Autodesk Inventor part; units mm, degrees
ref_plane "YZ Plane" through (0, 0, 0) normal (1, 0, 0) x (0, 1, 0)
ref_plane "XZ Plane" through (0, 0, 0) normal (0, 1, 0) x (-1, 0, 0)
ref_plane "XY Plane" through (0, 0, 0) normal (0, 0, 1) x (1, 0, 0)
sketch "Esboço1" plane through (0, 0, 0) normal (0, 1, 0) x (-1, 0, 0)
  line L0 (0, 0) -> (40, 0)
  line L1 (40, 0) -> (40, -60)
  line L2 (40, -60) -> (0, -60)
  line L3 (0, -60) -> (0, 0)
  dimension "d0" = 40
  dimension "d1" = 60
extrude "Extrusão1" add sketch "Esboço1" along normal blind 5
chamfer "Chanfro1" distance 3 angle 45 4 edges at (0, 2.5, 0) (-40, 2.5, 0) (0, 2.5, -60) (-40, 2.5, -60)
sketch "Esboço2" plane through (0, 5, 0) normal (0, 1, 0) x (1, 0, 0)
  line L0 (-3, 60) -> (-37, 60) construction
  line L1 (-20, 60) -> (-20, 0) construction
  line L2 (-20, 30) -> (0, 30) construction
  line L3 (-3, 30) -> (-3, 50) construction
  line L4 (-3, 30) -> (-3, 10) construction
  line L5 (0, 3) -> (0, 57)
  line L6 (0, 10) -> (-20, 10)
  line L7 (-20, 10) -> (-20, 13)
  line L8 (-20, 13) -> (0, 13)
  line L9 (0, 13) -> (0, 10)
  line L10 (0, 50) -> (-20, 50)
  line L11 (-20, 50) -> (-20, 47)
  line L12 (-20, 47) -> (0, 47)
  line L13 (0, 47) -> (0, 50)
  point P0 (0, 0)
  dimension "d7" = 20
  dimension "d8" = 20
  dimension "d9" = 3
  dimension "d10" = 3
extrude "Extrusão2" add sketch "Esboço2" along normal blind 20
chamfer "Chanfro2" distance 7 angle 45 4 edges at (-20, 25, -11.5) (0, 25, -11.5) (0, 25, -48.5) (-20, 25, -48.5)
sketch "Esboço3" plane through (0, 5, -13) normal (0, 0, -1) x (-1, 0, 0)
  line L0 (0, 13) -> (20, 13) construction
  line L1 (0, 13) -> (20, 13) construction
  line L2 (10, 13) -> (10, 20) construction
  line L3 (13, 20) -> (7, 20) construction
  circle A0 centre (10, 16.5) radius 2
  point P0 (0, -5)
  dimension "d16" = 4
extrude "Extrusão3" cut sketch "Esboço3" against normal blind 20
sketch "Esboço4" plane through (-20, 5, -47) normal (0, 0, 1) x (1, 0, 0)
  line L0 (0, 0) -> (0, 13) construction
  line L1 (20, 0) -> (20, 13) construction
  line L2 (0, 13) -> (20, 13) construction
  line L3 (20, 13) -> (10, 13) construction
  line L4 (10, 13) -> (10, 20) construction
  line L5 (13, 20) -> (7, 20) construction
  circle A0 centre (10, 16.5) radius 2
  point P0 (20, -5)
  dimension "d19" = 4
extrude "Extrusão4" cut sketch "Esboço4" against normal blind 666
chamfer "Chanfro3" distance 2 angle 45 9 edges at (-20, 5, -60) (-38.5, 5, -58.5) (-40, 5, -30) (-38.5, 5, -1.5) (-20, 5, 0) (-1.5, 5, -1.5) (0, 5, -6.5) (0, 5, -53.5) (-1.5, 5, -58.5)
sketch "Esboço5" plane through (0, 5, 0) normal (0, 1, 0) x (1, 0, 0)
  line L0 (0, 57) -> (0, 3)
  line L1 (0, 17.5) -> (-20, 17.5)
  line L2 (-20, 17.5) -> (-20, 42.5)
  line L3 (-20, 42.5) -> (0, 42.5)
  line L4 (0, 42.5) -> (0, 17.5)
  line L5 (-7, 13) -> (-13, 13)
  point P0 (0, 0)
  dimension "d25" = 20
  dimension "d26" = 25
  dimension "d27" = 4.5
extrude "Extrusão5" cut sketch "Esboço5" against normal blind 3
chamfer "Chanfro4" distance 3 angle 45 3 edges at (-20, 5, -30) (-10, 5, -42.5) (-10, 5, -17.5)
properties part number "Pezotta"
Build history of the part. All positions in model axes, mm. A direction names the side the tool comes from. Coordinates: 2 decimals unless noted, no trailing zeros. Order: outer loops, then holes, each group sorted by start corner. A loop starts at its lowest first (then second) coordinate and runs counter-clockwise, first axis right, second up. Notation, with made-up numbers: (54, -12.5) -> (60, -12.5) arc R28 cw to (60, 13.5) -> close; hole circle Ø1 at (70.25, 23). An arc over 180 degrees is marked (long way). One line per item, written item: value.
(1) Slice it at A-A, the plane y = 21.5. List the corners of the cut face in (x, z), plus the area to 3 significant figures.
Checked values:
outline: (-16.5, -50) -> (-12, -50) -> (-12, -47) -> (-16.5, -47) -> close; (-16.5, -13) -> (-12, -13) -> (-12, -10) -> (-16.5, -10) -> close; (-8, -50) -> (-3.5, -50) -> (-3.5, -47) -> (-8, -47) -> close; (-8, -13) -> (-3.5, -13) -> (-3.5, -10) -> (-8, -10) -> close
area: 54.0 mm2
(2) Tool access for faces 4 (the flat face through (-1, 4, -53)), 5 (the flat face through (-21, 3, -30)), 6 (the flat face through (-10, 13, -47)): list every direction of +Z, -Z, +X, -X, +Y, -Y with a clear straight run to the whole face (end or side of a thin tool).
Checked values:
face 4: -Z, +X, +Y
face 5: +X, +Y
face 6: +X, -X, +Y
(3) Mould opens along X. For faces 1 (the flat face through (-10, 2, -30)), 2 (the flat face through (-39, 1, -2)), 3 (the cylindrical face through (-11.474, 22.852, -48.479)) say: pulls with the +X half, pulls with the -X half, needs draft (parallel to the pull), parting line crosses it, or undercut.
Checked values:
face 1: needs draft
face 2: pulls with the -X half
face 3: undercut
(4) Slice it at B-B, the plane x = -10. Count the separate pieces of the cut face and the enclosed holes in it, plus the area to 3 significant figures.
Checked values:
separate pieces: 3
enclosed holes: 0
area: 308 mm2
(5) Probe line 1 (Z direction, x = -19.5, y = 17.75); line 2 (Y direction, x = -10, z = -47.7); line 3 (Y direction, x = -9, z = -54). List the from-to ranges inside material, lowest first. Write a range as [from, to].
Checked values:
line 1: [-50, -47], [-13, -10]
line 2: [0, 19.5], [23.5, 25]
line 3: [0, 5]
(6) Drop flat-ended pins along their axis: pin 1 Ø3.5 at (y, z) = (10.5, -48.5) entering from -X; pin 2 Ø10 at (x, y) = (-6.5, 16) entering from -Z; pin 3 Ø1.5 at (y, z) = (22.5, -14.5) entering from +X; pin 4 Ø6 at (x, y) = (-6, 12) entering from +Z. Give the stop position or say it passes through.
Checked values:
pin 1: x = -20
pin 2: z = -50
pin 3: through
pin 4: z = -10
